For this review, take the finished solid that the model builds, in its own axes (mm). A direction names the side the tool comes from. Give positions to 0.01 mm unless a question says otherwise; leave off trailing zeros. Order: outer loops, then holes, each group sorted by start corner. A loop starts at its lowest first (then second) coordinate and runs counter-clockwise, first axis right, second up. Notation, with made-up numbers: (-1, 0.5) - (8, 0.5) arc R18 ccw to (8, 25.5) - close; hole circle Ø11 at (69, -39). An arc over 180 degrees is marked (long way). One line per item, written item: value.
```python
from build123d import *

# Parameters (mm, degrees)
ESQUISSE2_W             = 35.2
ESQUISSE2_H             = 35.2
BOSS_EXTRU_1_DEPTH      = 28
ESQUISSE3_R             = 11
BOSS_EXTRU_2_DEPTH      = 2
ESQUISSE4_R             = 2.5
BOSS_EXTRU_3_DEPTH      = 24
ENL_V_MAT_EXTRU_1_DEPTH = 15
CHANFREIN1_SIZE         = 2
ESQUISSE6_R             = 1.5
ENL_V_MAT_EXTRU_2_DEPTH = 4.5


with BuildPart() as part:
    # Esquisse2 → Boss.-Extru.1 (new body)
    with BuildSketch(Plane.XY):
        with Locations((17.6, 17.6)):
            Rectangle(ESQUISSE2_W, ESQUISSE2_H)
    extrude(amount=BOSS_EXTRU_1_DEPTH)

    # Esquisse3 → Boss.-Extru.2 (add)
    with BuildSketch(Plane.XY.offset(28)):
        with Locations((17.6, 17.6)):
            Circle(ESQUISSE3_R)
    extrude(amount=BOSS_EXTRU_2_DEPTH)

    # Esquisse4 → Boss.-Extru.3 (add)
    with BuildSketch(Plane.XY.offset(30)):
        with Locations((17.6, 17.6)):
            Circle(ESQUISSE4_R)
    extrude(amount=BOSS_EXTRU_3_DEPTH)

    # Esquisse5 → Enl_v. mat.-Extru.1 (cut)
    with BuildSketch(Plane.XY.offset(54)):
        with BuildLine():
            Line((19.6, 19.1), (19.6, 16.1))
            ThreePointArc((19.6, 16.1), (20.1, 17.6), (19.6, 19.1))
        make_face()
    extrude(amount=-ENL_V_MAT_EXTRU_1_DEPTH, mode=Mode.SUBTRACT)

    # Chanfrein1
    chanfrein1_edges = [part.edges().sort_by_distance(p)[0] for p in [
        (0, 35.2, 14),
        (35.2, 35.2, 14),
        (35.2, 0, 14),
        (0, 0, 14),
    ]]
    chamfer(chanfrein1_edges, length=CHANFREIN1_SIZE)

    # Esquisse6 → Enl_v. mat.-Extru.2 (cut)
    with BuildSketch(Plane.XY.offset(28)):
        with Locations((30.6, 30.6)):
            Circle(ESQUISSE6_R)
        with Locations((30.6, 4.6)):
            Circle(ESQUISSE6_R)
        with Locations((4.6, 4.6)):
            Circle(ESQUISSE6_R)
        with Locations((4.6, 30.6)):
            Circle(ESQUISSE6_R)
    extrude(amount=-ENL_V_MAT_EXTRU_2_DEPTH, mode=Mode.SUBTRACT)


solid = part.part
```
(1) Take a section at A-A (y = 17.6). Write out the cut boundary in (x, z).
Answers below:
outline: (0, 0) - (35.2, 0) - (35.2, 28) - (28.6, 28) - (28.6, 30) - (20.1, 30) - (20.1, 39) - (19.6, 39) - (19.6, 54) - (15.1, 54) - (15.1, 30) - (6.6, 30) - (6.6, 28) - (0, 28) - close
(2) Draft analysis for pull direction Y (two halves, no side actions). For faces 1 (the face through (31, 31, 23.5)), 2 (the face through (5.986, 4.025, 25.782)), 3 (the face through (15.1, 17.7, 41.8)), 4 (the face through (1, 34.2, 13.8)), state which applies: pulls with the +Y half, pulls with the -Y half, needs draft (parallel to the pull), parting line crosses it, or undercut.
Answers below:
face 1: undercut
face 2: undercut
face 3: parting line crosses it
face 4: pulls with the +Y half
(3) Take a section at B-B (x = 17.6). Write out the cut boundary in (y, z).
Answers below:
outline: (0, 0) - (35.2, 0) - (35.2, 28) - (28.6, 28) - (28.6, 30) - (20.1, 30) - (20.1, 54) - (15.1, 54) - (15.1, 30) - (6.6, 30) - (6.6, 28) - (0, 28) - close
(4) For P1, Ø0.6, axis at x = 20, y = 17.5, coming from the +Z side; P2, Ø3.5, axis at x = 31, y = 5, coming from the +Z side; P3, Ø3.5, axis at y = 18.5, z = 46, coming from the +X side; P4, Ø8, axis at y = 24.5, z = 42.5, coming from the -X side, all flat-tipped, find the tip position at first contact; note any pin that passes through.
Answers below:
P1: stops at z = 39
P2: stops at z = 28
P3: stops at x = 19.6
P4: passes through
(5) Wall thickness on line 1 (Y direction, x = 30.6, z = 27); line 2 (X direction, y = 30, z = 24); line 3 (Z direction, x = 26, y = 15.5): over which ranges is each line inside the solid? List them lowest first. Write a range as from..to.
Answers below:
line 1: y = 0..3.1, 6.1..29.1, 32.1..35.2
line 2: x = 0..3.23, 5.97..29.23, 31.97..35.2
line 3: z = 0..30
(6) Take a section at D-D (z = 47). Write out the cut boundary in (x, y), then the cut area to 3 significant figures.
Answers below:
outline: (19.6, 16.1) - (19.6, 19.1) arc R2.5 ccw (long way) to start
area: 18.6 mm^2
(7) Machinability: for faces 5 (the face through (19.6, 18, 47)), 6 (the face through (17, 18, 54)), 7 (the face through (31, 5, 23.5)), which of the approach directions +Z, -Z, +X, -X, +Y, -Y give a long, thin tool a straight path to every point of the face, cutting with its end or side? Answer none if there is none.
Answers below:
face 5: +Z, +X, +Y, -Y
face 6: +Z, +X, -X, +Y, -Y
face 7: +Z
(8) Take a section at C-C (y = 4.6). Write out the cut boundary in (x, z).
Answers below:
outline: (0, 0) - (35.2, 0) - (35.2, 28) - (32.1, 28) - (32.1, 23.5) - (29.1, 23.5) - (29.1, 28) - (6.1, 28) - (6.1, 23.5) - (3.1, 23.5) - (3.1, 28) - (0, 28) - close
